```python
from build123d import *

# Parameters (mm, degrees)
F1_DEPTH = 20
F3_DEPTH = 25
F4_R     = 30
F5_R     = 3
F6_R     = 3


with BuildPart() as f1:
    # F0 (on Top) → F1 (new body)
    with BuildSketch(Plane.XY):
        with BuildLine():
            Line((-100, -150), (100, -150))
            ThreePointArc((100, -150), (117.67767, -142.67767), (125, -125))
            Line((125, -125), (125, 125))
            ThreePointArc((125, 125), (117.67767, 142.67767), (100, 150))
            Line((100, 150), (-100, 150))
            ThreePointArc((-100, 150), (-117.67767, 142.67767), (-125, 125))
            Line((-125, 125), (-125, -125))
            ThreePointArc((-125, -125), (-117.67767, -142.67767), (-100, -150))
        make_face()
    extrude(amount=F1_DEPTH)

    # F2 (on face) → F3 (cut)
    with BuildSketch(Plane.XY.offset(20)):
        with BuildLine():
            Line((-48, -80), (-125, -80))
            Line((-125, -80), (-125, -125))
            ThreePointArc((-125, -125), (-117.67767, -142.67767), (-100, -150))
            Line((-100, -150), (-48, -150))
            Line((-48, -150), (-48, -80))
        make_face()
        with BuildLine():
            Line((-125, -80), (-146.106765, -80))
            Line((-146.106765, -80), (-146.106765, -176.229358))
            Line((-146.106765, -176.229358), (-48, -176.229358))
            Line((-48, -176.229358), (-48, -150))
            Line((-48, -150), (-100, -150))
            ThreePointArc((-100, -150), (-117.67767, -142.67767), (-125, -125))
            Line((-125, -125), (-125, -80))
        make_face()
        with BuildLine():
            Line((-146.106765, 80), (-125, 80))
            Line((-125, 80), (-125, 125))
            ThreePointArc((-125, 125), (-117.67767, 142.67767), (-100, 150))
            Line((-100, 150), (-48, 150))
            Line((-48, 150), (-48, 176.229358))
            Line((-48, 176.229358), (-146.106765, 176.229358))
            Line((-146.106765, 176.229358), (-146.106765, 80))
        make_face()
        with BuildLine():
            Line((-125, 125), (-125, 80))
            Line((-125, 80), (-48, 80))
            Line((-48, 80), (-48, 150))
            Line((-48, 150), (-100, 150))
            ThreePointArc((-100, 150), (-117.67767, 142.67767), (-125, 125))
        make_face()
    extrude(amount=-F3_DEPTH, mode=Mode.SUBTRACT)

    # F4
    f4_edges = [f1.edges().sort_by_distance(p)[0] for p in [
        (-48, -150, 10),
        (-48, 150, 10),
    ]]
    fillet(f4_edges, radius=F4_R)

    # F5
    f5_edges = [f1.edges().sort_by_distance(p)[0] for p in [
        (-48, 80, 10),
        (-125, 80, 10),
        (-48, -80, 10),
        (-125, -80, 10),
    ]]
    fillet(f5_edges, radius=F5_R)

    # F6
    f6_edges = [f1.edges().sort_by_distance(p)[0] for p in [
        (-48, 101.5, 20),
        (-48.87868, 80.87868, 20),
        (-39.213203, 141.213203, 20),
        (-86.5, 80, 20),
        (41, 150, 20),
        (-124.12132, 79.12132, 20),
        (117.67767, 142.67767, 20),
        (-125, 0, 20),
        (125, 0, 20),
        (-124.12132, -79.12132, 20),
        (117.67767, -142.67767, 20),
        (-86.5, -80, 20),
        (41, -150, 20),
        (-48.87868, -80.87868, 20),
        (-39.213203, -141.213203, 20),
        (-48, -101.5, 20),
        (-48, 101.5, 0),
        (-48.87868, 80.87868, 0),
        (-39.213203, 141.213203, 0),
        (-86.5, 80, 0),
        (41, 150, 0),
        (-124.12132, 79.12132, 0),
        (117.67767, 142.67767, 0),
        (-125, 0, 0),
        (125, 0, 0),
        (-124.12132, -79.12132, 0),
        (117.67767, -142.67767, 0),
        (-86.5, -80, 0),
        (41, -150, 0),
        (-48.87868, -80.87868, 0),
        (-39.213203, -141.213203, 0),
        (-48, -101.5, 0),
    ]]
    fillet(f6_edges, radius=F6_R)


solid = f1.part
```
For this review, take the finished solid that the model builds, in its own axes (mm). A direction names the side the tool comes from. Round coordinates to 2 decimals unless told otherwise and drop trailing zeros. Write each loop counter-clockwise with the first axis right and the second up, starting at its lowest first coordinate (ties: lowest second). Pieces come first, ordered by that corner, then holes. Notation, with made-up numbers: (-36.75, -31.5) -> (-18.75, -31.5) arc R9 ccw to (-18.75, -26.5) -> close; hole circle Ø2 at (-15.5, 74). An arc over 180 degrees is marked (long way). Use one line per item in the form item = value.
Q1. Consider section C-C (y = -89). State the section outline as (x, z) points.
Resolved:
outline = (-48, 3) arc R3 ccw to (-45, 0) -> (122, 0) arc R3 ccw to (125, 3) -> (125, 17) arc R3 ccw to (122, 20) -> (-45, 20) arc R3 ccw to (-48, 17) -> close
Q2. Consider section A-A (z = 11.75). State the section outline as (x, y) points.
Resolved:
outline = (-125, -77) arc R3 ccw to (-122, -80) -> (-51, -80) arc R3 cw to (-48, -83) -> (-48, -120) arc R30 ccw to (-18, -150) -> (100, -150) arc R25 ccw to (125, -125) -> (125, 125) arc R25 ccw to (100, 150) -> (-18, 150) arc R30 ccw to (-48, 120) -> (-48, 83) arc R3 cw to (-51, 80) -> (-122, 80) arc R3 ccw to (-125, 77) -> close
Q3. To check wall thickness, follow probe 1 along X at (y, z) = (-92.5, 10.75); probe 2 along Y at (x, z) = (-54, 13.75); probe 3 along X at (y, z) = (-40.5, 17.5). State the ranges of each line that lie inside material, in increasing order. Write a range as from..to.
Resolved:
probe_1 = -48..125
probe_2 = -80..80
probe_3 = -124.96..124.96
Q4. Clearance check with flat-ended pins moving along their axes: pin 1 Ø11 at (x, z) = (-84.5, 9.5) entering from +Y; pin 2 Ø4 at (y, z) = (98.5, 12.5) entering from -X; pin 3 Ø4 at (x, z) = (-104, 9.5) entering from -Y. State where each tip first meets the part, or that it passes through.
Resolved:
pin_1 = 80
pin_2 = -48
pin_3 = -80
Q5. Consider section B-B (x = -59.5). State the section outline as (y, z) points, then the cut area to 3 significant figures.
Resolved:
outline = (-80, 3) arc R3 ccw to (-77, 0) -> (77, 0) arc R3 ccw to (80, 3) -> (80, 17) arc R3 ccw to (77, 20) -> (-77, 20) arc R3 ccw to (-80, 17) -> close
area = 3,190 mm²
Q6. Machinability: for faces 1 (the flat face through (-48, -102, 10)), 2 (the flat face through (-87, 80, 10)), 3 (the cylindrical face through (117.871, 142.482, 9.902)), which of the approach directions +Z, -Z, +X, -X, +Y, -Y give a long, thin tool a straight path to every point of the face, cutting with its end or side? Answer none if there is none.
Resolved:
face_1 = +Z, -Z, -X, -Y
face_2 = +Z, -Z, -X, +Y
face_3 = +Z, -Z, +X, +Y
